The listing builds one solid part. Answer for the finished solid, in the listing's coordinates (mm). Face numbers are marked on the shaded views. A direction names the side the tool comes from. Give positions to 0.01 mm unless a question says otherwise; leave off trailing zeros. Write each loop counter-clockwise with the first axis right and the second up, starting at its lowest first coordinate (ties: lowest second). Pieces come first, ordered by that corner, then holes. Notation, with made-up numbers: (67, -4.75) - (110, -4.75) arc R34 cw to (110, 27.25) - close; hole circle Ø11 at (36, 77.25). An arc over 180 degrees is marked (long way). One line per item, written item: value. Start each with the question number.
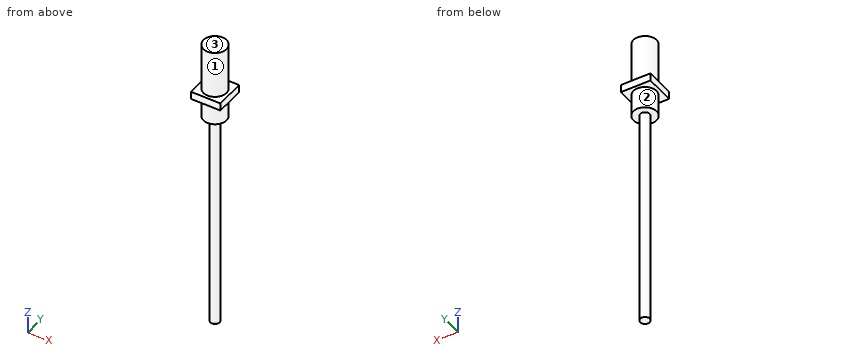
from build123d import *

# Parameters (mm, degrees)
SKETCH1_R           = 1.016
BOSS_EXTRUDE1_DEPTH = 47.371
BOSS_EXTRUDE2_START = 0.0254
SKETCH2_R           = 1.016
BOSS_EXTRUDE2_DEPTH = 0.0254
SKETCH3_W           = 1.27
SKETCH3_H           = 1.27
BOSS_EXTRUDE3_DEPTH = 0.0254
BOSS_EXTRUDE4_START = 0.0254
SKETCH4_R           = 1.016
BOSS_EXTRUDE4_DEPTH = 0.0254
SKETCH5_R           = 2.4892
BOSS_EXTRUDE5_DEPTH = 4.699
SKETCH6_W           = 6.35
SKETCH6_H           = 6.35
BOSS_EXTRUDE6_DEPTH = 1.651
SKETCH7_R           = 2.4892
BOSS_EXTRUDE7_DEPTH = 10.16


with BuildPart() as part:
    # Sketch1 → Boss-Extrude1 (new body)
    with BuildSketch(Plane.XY):
        Circle(SKETCH1_R)
    extrude(amount=BOSS_EXTRUDE1_DEPTH)

    # Sketch2 → Boss-Extrude2 (add)
    with BuildSketch(Plane(origin=(0, 0, 0), x_dir=(-1, 0, 0), z_dir=(0, 0, -1)).offset(BOSS_EXTRUDE2_START)):
        Circle(SKETCH2_R)
    extrude(amount=-BOSS_EXTRUDE2_DEPTH)

    # Sketch3 → Boss-Extrude3 (add)
    with BuildSketch(Plane(origin=(0, 0, -0.0254), x_dir=(-1, 0, 0), z_dir=(0, 0, -1))):
        Rectangle(SKETCH3_W, SKETCH3_H)
    extrude(amount=BOSS_EXTRUDE3_DEPTH)

    # Sketch4 → Boss-Extrude4 (add)
    with BuildSketch(Plane(origin=(0, 0, -0.0508), x_dir=(-1, 0, 0), z_dir=(0, 0, -1)).offset(BOSS_EXTRUDE4_START)):
        Circle(SKETCH4_R)
    extrude(amount=-BOSS_EXTRUDE4_DEPTH)

    # Sketch5 → Boss-Extrude5 (add)
    with BuildSketch(Plane.XY.offset(47.371)):
        Circle(SKETCH5_R)
    extrude(amount=BOSS_EXTRUDE5_DEPTH)

    # Sketch6 → Boss-Extrude6 (add)
    with BuildSketch(Plane.XY.offset(52.07)):
        Rectangle(SKETCH6_W, SKETCH6_H)
    extrude(amount=BOSS_EXTRUDE6_DEPTH)

    # Sketch7 → Boss-Extrude7 (add)
    with BuildSketch(Plane.XY.offset(53.721)):
        Circle(SKETCH7_R)
    extrude(amount=BOSS_EXTRUDE7_DEPTH)


solid = part.part
Item 1: Find section C-C on z = 46. Determine the outline of the cut face in (x, y), plus the area to 3 significant figures.
Item 2: Find section A-A on y = 0. Determine the outline of the cut face in (x, z) (3 decimals), plus the area to 3 significant figures.
Item 3: For the marked faces 1, 2 and 3, determine the directions among +Z, -Z, +X, -X, +Y, -Y from which every point of the face is accessible in a straight line to the end or side of a thin tool.
Item 4: Straight lines are drawn through the part: line 1 along Z through (x, y) = (1, -2); line 2 along Z through (x, y) = (2.5, -2); line 3 along Y through (x, z) = (-0.75, 39). For each, find the intervals that lie inside material, in ascending order.
Item 5: Each of these flat-tipped pins is pushed along its axis until it touches: pin 1 Ø2 at (y, z) = (-1, 19.5) entering from -X; pin 2 Ø1.5 at (x, y) = (-2, -0.5) entering from -Z. Where does it stop, or does it pass through?
Values:
1. outline: circle Ø2.03 at (0, 0)
1. area: 3.24 mm^2
2. outline: (-3.175, 52.07) - (-2.489, 52.07) - (-2.489, 47.371) - (-1.016, 47.371) - (-1.016, -0.025) - (-0.635, -0.025) - (-0.635, -0.051) - (-1.016, -0.051) - (-1.016, -0.076) - (1.016, -0.076) - (1.016, -0.051) - (0.635, -0.051) - (0.635, -0.025) - (1.016, -0.025) - (1.016, 47.371) - (2.489, 47.371) - (2.489, 52.07) - (3.175, 52.07) - (3.175, 53.721) - (2.489, 53.721) - (2.489, 63.881) - (-2.489, 63.881) - (-2.489, 53.721) - (-3.175, 53.721) - close
2. area: 181 mm^2
3. face 1: +Z
3. face 2: -Z
3. face 3: +Z, +X, -X, +Y, -Y
4. line 1: 47.37 to 63.88
4. line 2: 52.07 to 53.72
4. line 3: -0.69 to 0.69
5. pin 1: x = -1.02
5. pin 2: z = 47.37
